Verification items for the finished model (mm, model axes). A direction names the side the tool comes from. Coordinates: 2 decimals unless noted, no trailing zeros. Loops run counter-clockwise (first coordinate to the right, second up) from the corner with the lowest first, then second, coordinate; pieces in that order, holes last.
Q1. Material ranges on probe 1 along Y at (x, z) = (0, 8.75); probe 2 along Z at (x, y) = (14, 25); probe 3 along X at (y, z) = (21, 5), recorded low to high.
Q2. Sectioned sample at B-B (z = 5). Enter the section's corners in (x, y).
Q3. Go/stop test with flat-tipped pins: P1, Ø3, axis at x = 15, z = 2.5, coming from the +Y side; P2, Ø4, axis at x = -5, z = 5.5, coming from the +Y side; P3, Ø4.5, axis at x = -14, z = 5, coming from the +Y side; P4, Ø6, axis at x = -13, z = 5.5, coming from the +Y side. Record where each tip stops, or that it passes through.
Q4. Sectioned sample at C-C (x = 0). Enter the section's corners in (y, z).
Q5. Sectioned sample at D-D (y = 8). Enter the section's corners in (x, z).
Q6. Sectioned sample at A-A (y = 25). Enter the section's corners in (x, z).
Q7. Mould release check, pull along Z, two halves, no side actions. Record for faces 1 (the face through (-7.552, 44.146, 5.063)), 2 (the face through (-14.995, 36.759, 0.254)), 3 (the face through (-11.33, 25.92, 4.16)), 4 (the face through (15.433, 4.93, 4.086)): +Z half, -Z half, draft (parallel to the pull), parting line (faces both ways), or undercut.
Q8. Access from +Z, -Z, +X, -X, +Y, -Y to the whole of each face (thin tool, end or side, straight path). Record for faces 5 (the face through (11.2, 26, 4.9)), 6 (the face through (17.19, 34.66, 4.94)).
```python
from build123d import *

# Parameters (mm, degrees)
SKETCH1_R            = 8.25
BOSS_EXTRUDE1_DEPTH  = 10
M3_CLEARANCE_HOLE1_D = 3.4
SKETCH2_R            = 2.8
CUT_EXTRUDE1_DEPTH   = 35
FILLET1_R            = 10
FILLET2_R            = 2
CHAMFER1_SIZE        = 0.5


with BuildPart() as part:
    # Sketch1 → Boss-Extrude1 (new body)
    with BuildSketch(Plane.XY):
        Polygon((8, 45), (-8, 45), (-20, 31.5), (-20, 0), (20, 0), (20, 31.5), align=None)
        with Locations((0, 25)):
            Circle(SKETCH1_R, mode=Mode.SUBTRACT)
    extrude(amount=BOSS_EXTRUDE1_DEPTH)

    # M3 Clearance Hole1 (through all)
    with Locations(Plane(origin=(-14, 45, 5), x_dir=(0, 0, 1), z_dir=(0, 1, 0))):
        with Locations((0, 0), (0, 28)):
            Hole(M3_CLEARANCE_HOLE1_D / 2)

    # Sketch2 → Cut-Extrude1 (cut)
    with BuildSketch(Plane(origin=(0, 45, 0), x_dir=(1, 0, 0), z_dir=(0, 1, 0))):
        with Locations((14, -5)):
            Circle(SKETCH2_R)
        with Locations((-14, -5)):
            Circle(SKETCH2_R)
    extrude(amount=-CUT_EXTRUDE1_DEPTH, mode=Mode.SUBTRACT)

    # Fillet1
    fillet1_edges = [part.edges().sort_by_distance(p)[0] for p in [
        (-8, 45, 5),
        (8, 45, 5),
    ]]
    fillet(fillet1_edges, radius=FILLET1_R)

    # Fillet2
    fillet2_edges = [part.edges().sort_by_distance(p)[0] for p in [
        (-20, 31.5, 5),
        (20, 31.5, 5),
    ]]
    fillet(fillet2_edges, radius=FILLET2_R)

    # Chamfer1
    chamfer1_edges = [part.edges().sort_by_distance(p)[0] for p in [
        (-15.239125591, 36.855983711, 0),
        (-15.239125591, 36.855983711, 10),
        (0, 45, 0),
        (15.239125591, 36.855983711, 0),
        (7.605899873, 44.122400558, 0),
        (-7.605899873, 44.122400558, 0),
        (0, 45, 10),
        (15.239125591, 36.855983711, 10),
        (7.605899873, 44.122400558, 10),
        (-7.605899873, 44.122400558, 10),
        (-20, 15.369800678, 0),
        (-20, 15.369800678, 10),
        (20, 15.369800678, 0),
        (19.869443403, 31.45036247, 0),
        (-19.869443403, 31.45036247, 0),
        (20, 15.369800678, 10),
        (19.869443403, 31.45036247, 10),
        (-19.869443403, 31.45036247, 10),
    ]]
    chamfer(chamfer1_edges, length=CHAMFER1_SIZE)


solid = part.part
```
Geometry check:
1. probe 1: y = 0 to 16.75, 33.25 to 45
1. probe 2: z = 0 to 2.2, 7.8 to 10
1. probe 3: x = -20 to -16.8, -11.2 to -7.22, 7.22 to 11.2, 16.8 to 20
2. outline: (-20, 0) - (-15.7, 0) - (-15.7, 10) - (-16.8, 10) - (-16.8, 35.1) - (-19.49, 32.07) arc R2 ccw to (-20, 30.74) - close; (-12.3, 0) - (12.3, 0) - (12.3, 10) - (11.2, 10) - (11.2, 41.4) - (10.98, 41.64) arc R10 ccw to (3.51, 45) - (-3.51, 45) arc R10 ccw to (-10.98, 41.64) - (-11.2, 41.4) - (-11.2, 10) - (-12.3, 10) - close; (15.7, 0) - (20, 0) - (20, 30.74) arc R2 ccw to (19.49, 32.07) - (16.8, 35.1) - (16.8, 10) - (15.7, 10) - close; hole circle Ø16.5 at (0, 25)
3. P1: stops at y = 38.79
3. P2: stops at y = 45
3. P3: stops at y = 10
3. P4: stops at y = 42.61
4. outline: (0, 0) - (16.75, 0) - (16.75, 10) - (0, 10) - close; (33.25, 0) - (44.5, 0) - (45, 0.5) - (45, 9.5) - (44.5, 10) - (33.25, 10) - close
5. outline: (-20, 0.5) - (-19.5, 0) - (19.5, 0) - (20, 0.5) - (20, 9.5) - (19.5, 10) - (-19.5, 10) - (-20, 9.5) - close; hole circle Ø3.4 at (-14, 5); hole circle Ø3.4 at (14, 5)
6. outline: (-20, 0.5) - (-19.5, 0) - (-8.25, 0) - (-8.25, 10) - (-19.5, 10) - (-20, 9.5) - close; (8.25, 0) - (19.5, 0) - (20, 0.5) - (20, 9.5) - (19.5, 10) - (8.25, 10) - close; hole circle Ø5.6 at (-14, 5); hole circle Ø5.6 at (14, 5)
7. face 1: draft
7. face 2: -Z half
7. face 3: undercut
7. face 4: undercut
8. face 5: +Y
8. face 6: +Z, -Z, +X, +Y
